```python
from build123d import *

# Parameters (mm, degrees)
F1_DEPTH = 6.5
F2_DEPTH = 3.5
F3_DEPTH = 25
F4_R     = 3.49999
F5_SIZE2 = 15
F5_SIZE  = 5
F6_R     = 4


# Not quite as in the source:
# - a fillet or chamfer is up to 0.001 mm smaller than in the source, because OpenCascade refuses the exact size


with BuildPart() as f1:
    # F0 (on Top) → F1 (new body)
    with BuildSketch(Plane.XY):
        with BuildLine():
            Line((-1.6568542495, 1.6568542495), (-1.6568542495, 30))
            Line((-1.6568542495, 30), (-11.6568542495, 30))
            ThreePointArc((-11.6568542495, 30), (-17.0460019087, 17.0460019087), (-30, 11.6568542495))
            Line((-30, 11.6568542495), (-30, 1.6568542495))
            Line((-30, 1.6568542495), (-1.6568542495, 1.6568542495))
        make_face()
    extrude(amount=F1_DEPTH)

    # F0 (on Top) → F2 (join)
    with BuildSketch(Plane.XY):
        Polygon((24.3431457505, -24.3431457505), (24.3431457505, 30), (-1.6568542495, 30), (-1.6568542495, 1.6568542495), (-30, 1.6568542495), (-30, -24.3431457505), align=None)
    extrude(amount=F2_DEPTH)

    # F0 (on Top) → F3 (join)
    with BuildSketch(Plane.XY):
        with BuildLine():
            ThreePointArc((-30, -24.3431457505), (30, -30), (24.3431457505, 30))
            Line((24.3431457505, 30), (24.3431457505, -24.3431457505))
            Line((24.3431457505, -24.3431457505), (-30, -24.3431457505))
        make_face()
    extrude(amount=F3_DEPTH)

    # F4 (radius 3.5 in the source; OpenCascade refuses exactly that, so slightly less here)
    f4_edges = [f1.edges().sort_by_distance(p)[0] for p in [
        (30, -30, 0),
        (-30, -6.343146, 0),
        (6.343146, 30, 0),
    ]]
    fillet(f4_edges, radius=F4_R)

    # F5
    f5_edges = [f1.edges().sort_by_distance(p)[0] for p in [
        (30, -30, 25),
    ]]
    f5_side = f1.faces().sort_by_distance((29.285433, -29.285433, 25))[0]
    chamfer(f5_edges, length=F5_SIZE, length2=F5_SIZE2, reference=f5_side)

    # F6
    f6_edges = [f1.edges().sort_by_distance(p)[0] for p in [
        (26.464466, -26.464466, 25),
    ]]
    fillet(f6_edges, radius=F6_R)


solid = f1.part
```
Part model, mm, in its own coordinate system. A direction names the side the tool comes from. Coordinates: 2 decimals unless noted, no trailing zeros. Order: outer loops, then holes, each group sorted by start corner. A loop starts at its lowest first (then second) coordinate and runs counter-clockwise, first axis right, second up. Notation, with made-up numbers: (87, 56) - (106, 56) arc R26 cw to (106, 75) - close; hole circle Ø11 at (52, -17). An arc over 180 degrees is marked (long way). Return JSON: item names as keys, results as strings. Group by question number.
Item 1: Pull direction X, two halves, no side cores. Call faces 3 (the face through (-1.657, 16, 5)), 4 (the face through (3, -3, 3.5)), 5 (the face through (-16, 1.657, 5)), 6 (the face through (29.311, -30.673, 6.704)): pulls with the +X half, pulls with the -X half, needs draft (parallel to the pull), parting line crosses it, or undercut.
Item 2: Pin check, flat tips, straight feed: pin 1 (4 mm diameter, centred on x = -21.5, z = 10, fed in from -Y); pin 2 (3 mm diameter, centred on y = -25.5, z = 14.5, fed in from -X); pin 3 (1.5 mm diameter, centred on y = 8.5, z = 22, fed in from +X). Stop position of each tip, or through.
Item 3: Drill centre lines: probe 1 along Z at (x, y) = (-21, 9.5); probe 2 along Z at (x, y) = (-3.5, -12.5); probe 3 along X at (y, z) = (-33, 4.5). Where is each one in solid material? Low to high. Write a range as from..to.
Item 4: Cut at B-B (z = 18). List the corners of the cut face in (x, y), plus the area to 3 significant figures.
Item 5: Cut at A-A (z = 5). List the corners of the cut face in (x, y).
Item 6: Cut at C-C (z = 11.25). List the corners of the cut face in (x, y), plus the area to 3 significant figures.
Item 7: Which spindle directions (+Z, -Z, +X, -X, +Y, -Y) get a long thin tool onto all of the face, cutting with end or side? Do faces 1 (the face through (-13, 13, 6.5)), 2 (the face through (5, -5, 0)). Say none if no direction does.
Check values:
{
 "1": {"face 3": "undercut", "face 4": "undercut", "face 5": "needs draft", "face 6": "parting line crosses it"},
 "2": {"pin 1": "stops at y = -34.79", "pin 2": "stops at x = -28.56", "pin 3": "stops at x = 36.09"},
 "3": {"probe 1": "z = 0..6.5", "probe 2": "z = 0..3.5", "probe 3": "x = -21.95..26.63"},
 "4": {"outline": "(-26.72, -24.34) arc R36.45 ccw (long way) to (24.34, 26.72) - (24.34, -24.34) - close", "area": "1,150 mm2"},
 "5": {"outline": "(-30, -24.34) arc R39.12 ccw (long way) to (24.34, 30) - (24.34, -24.34) - close; (-30, 1.66) - (-1.66, 1.66) - (-1.66, 30) - (-11.66, 30) arc R18.4 cw to (-30, 11.66) - close"},
 "6": {"outline": "(-29.49, -24.34) arc R38.7 ccw (long way) to (24.34, 29.49) - (24.34, -24.34) - close", "area": "1,440 mm2"},
 "7": {"face 1": "+Z, -X, +Y", "face 2": "-Z, +X, -X, +Y, -Y"}
}
